from build123d import *

# Parameters (mm, degrees)
BOSS_EXTRU_1_DEPTH                             = 84
FRAISAGE_POUR_VIS_T_TE_FRAIS_E_M31_D           = 3.2
FRAISAGE_POUR_VIS_T_TE_FRAIS_E_M31_DEPTH       = 4
FRAISAGE_POUR_VIS_T_TE_FRAIS_E_M31_CSINK_D     = 6.3
FRAISAGE_POUR_VIS_T_TE_FRAIS_E_M31_CSINK_ANGLE = 90
D_GAGEMENT_M1_61_D                             = 1.7
D_GAGEMENT_M1_61_DEPTH                         = 4
ENL_V_MAT_EXTRU_1_DEPTH                        = 4
ENL_V_MAT_EXTRU_2_DEPTH                        = 31.75
ENL_V_MAT_EXTRU_2_DEPTH_BACK                   = 5


with BuildPart() as part:
    # Esquisse1 → Boss.-Extru.1 (new body)
    with BuildSketch(Plane.XY):
        with BuildLine():
            Line((0, 0), (-25, 0))
            ThreePointArc((-25, 0), (-32.071067812, 2.928932188), (-35, 10))
            Line((-35, 10), (-35, 45))
            Line((-35, 45), (-31, 45))
            Line((-31, 45), (-31, 10))
            ThreePointArc((-31, 10), (-29.242640687, 5.757359313), (-25, 4))
            Line((-25, 4), (0, 4))
            Line((0, 4), (0, 0))
        make_face()
    extrude(amount=BOSS_EXTRU_1_DEPTH)

    # Fraisage pour vis à tête fraisée M31
    with Locations(Plane(origin=(-31, 0, 0), x_dir=(0, 0, 1), z_dir=(1, 0, 0))):
        with Locations((4, -41), (80, -41)):
            CounterSinkHole(FRAISAGE_POUR_VIS_T_TE_FRAIS_E_M31_D / 2, FRAISAGE_POUR_VIS_T_TE_FRAIS_E_M31_CSINK_D / 2, depth=FRAISAGE_POUR_VIS_T_TE_FRAIS_E_M31_DEPTH, counter_sink_angle=FRAISAGE_POUR_VIS_T_TE_FRAIS_E_M31_CSINK_ANGLE)

    # Dégagement M1.61
    with Locations(Plane(origin=(0, 0, 0), x_dir=(-1, 0, 0), z_dir=(0, -1, 0))):
        with Locations((20.75, -21.5), (20.75, -62.5), (4.25, -62.5), (4.25, -21.5)):
            Hole(D_GAGEMENT_M1_61_D / 2, depth=D_GAGEMENT_M1_61_DEPTH)

    # Esquisse6 → Enlèv. mat.-Extru.1 (cut)
    with BuildSketch(Plane.XZ):
        with BuildLine():
            Line((-35, 17.5), (-3.25, 17.5))
            ThreePointArc((-3.25, 17.5), (-1.128679656, 18.378679656), (-0.25, 20.5))
            Line((-0.25, 20.5), (-0.25, 23.5))
            ThreePointArc((-0.25, 23.5), (-0.835786438, 24.914213562), (-2.25, 25.5))
            Line((-2.25, 25.5), (-3.750142858, 25.5))
            ThreePointArc((-3.750142858, 25.5), (-5.097923909, 25.180202649), (-6.15836042, 24.288990826))
            ThreePointArc((-6.15836042, 24.288990826), (-17.832822404, 23.171534919), (-17.754587156, 34.899094322))
            ThreePointArc((-17.754587156, 34.899094322), (-17.012643745, 35.911706018), (-16.75, 37.139256723))
            Line((-16.75, 37.139256723), (-16.75, 46.860743277))
            ThreePointArc((-16.75, 46.860743277), (-17.012643745, 48.088293982), (-17.754587156, 49.100905678))
            ThreePointArc((-17.754587156, 49.100905678), (-17.832822404, 60.828465081), (-6.15836042, 59.711009174))
            ThreePointArc((-6.15836042, 59.711009174), (-5.097923909, 58.819797351), (-3.750142858, 58.5))
            Line((-3.750142858, 58.5), (-2.25, 58.5))
            ThreePointArc((-2.25, 58.5), (-0.835786438, 59.085786438), (-0.25, 60.5))
            Line((-0.25, 60.5), (-0.25, 63.5))
            ThreePointArc((-0.25, 63.5), (-1.128679656, 65.621320344), (-3.25, 66.5))
            Line((-3.25, 66.5), (-35, 66.5))
            Line((-35, 66.5), (-35, 84))
            Line((-35, 84), (0, 84))
            Line((0, 84), (0, 0))
            Line((0, 0), (-35, 0))
            Line((-35, 0), (-35, 17.5))
        make_face()
        with BuildLine():
            Line((-18.75, 46), (-18.75, 38))
            ThreePointArc((-18.75, 38), (-20.75, 36), (-22.75, 38))
            Line((-22.75, 38), (-22.75, 46))
            ThreePointArc((-22.75, 46), (-20.75, 48), (-18.75, 46))
        make_face()
    extrude(amount=-ENL_V_MAT_EXTRU_1_DEPTH, mode=Mode.SUBTRACT)

    # Esquisse7 → Enlèv. mat.-Extru.2 (cut, two sides)
    with BuildSketch(Plane(origin=(-31, 0, 0), x_dir=(0, 0, -1), z_dir=(1, 0, 0))) as enl_v_mat_extru_2_sk:
        with BuildLine():
            Line((-60.518790495, 10), (-23.481209505, 10))
            Line((-23.481209505, 10), (-17.352509418, 22.636031611))
            ThreePointArc((-17.352509418, 22.636031611), (-17.875393601, 32.308498663), (-26.350052411, 37))
            Line((-26.350052411, 37), (-57.649947589, 37))
            ThreePointArc((-57.649947589, 37), (-66.124606399, 32.308498663), (-66.647490582, 22.636031611))
            Line((-66.647490582, 22.636031611), (-60.518790495, 10))
        make_face()
        with BuildLine():
            Line((-23.657740647, 9.636031611), (-23.481209505, 10))
            Line((-23.481209505, 10), (-60.518790495, 10))
            Line((-60.518790495, 10), (-60.342259353, 9.636031611))
            ThreePointArc((-60.342259353, 9.636031611), (-56.653215023, 5.52534119), (-51.34471636, 4))
            Line((-51.34471636, 4), (-32.65528364, 4))
            ThreePointArc((-32.65528364, 4), (-27.346784977, 5.52534119), (-23.657740647, 9.636031611))
        make_face()
        Polygon((0, 4), (0, 10), (-14.589893279, 10), (-17.5, 4), align=None)
        with BuildLine():
            Line((0, 10), (0, 41))
            ThreePointArc((0, 41), (-0.101534354, 40.104474676), (-0.400982803, 39.254412644))
            Line((-0.400982803, 39.254412644), (-14.589893279, 10))
            Line((-14.589893279, 10), (0, 10))
        make_face()
        with BuildLine():
            ThreePointArc((-4, 45), (-1.171572875, 43.828427125), (0, 41))
            Line((0, 41), (0, 45))
            Line((0, 45), (-4, 45))
        make_face()
        with BuildLine():
            ThreePointArc((-83.599017197, 39.254412644), (-83.898465646, 40.104474676), (-84, 41))
            Line((-84, 41), (-84, 10))
            Line((-84, 10), (-69.410106721, 10))
            Line((-69.410106721, 10), (-83.599017197, 39.254412644))
        make_face()
        Polygon((-69.410106721, 10), (-84, 10), (-84, 4), (-66.5, 4), align=None)
        with BuildLine():
            ThreePointArc((-84, 41), (-82.828427125, 43.828427125), (-80, 45))
            Line((-80, 45), (-84, 45))
            Line((-84, 45), (-84, 41))
        make_face()
    extrude(amount=ENL_V_MAT_EXTRU_2_DEPTH, mode=Mode.SUBTRACT)
    extrude(enl_v_mat_extru_2_sk.sketch, amount=-ENL_V_MAT_EXTRU_2_DEPTH_BACK, mode=Mode.SUBTRACT)


solid = part.part
Input: part model. Units: mm. Frame: model coordinates. A direction names the side the tool comes from. Coordinates: 2 decimals unless noted, no trailing zeros. Loops run counter-clockwise (first coordinate to the right, second up) from the corner with the lowest first, then second, coordinate; pieces in that order, holes last.
(1) First-contact query: pin 1 Ø1.2 at (y, z) = (1, 43.5) entering from -X; pin 2 Ø3.5 at (y, z) = (41, 80) entering from +X; pin 3 Ø16.5 at (x, z) = (-10.5, 30.5) entering from +Y. Flat tips, straight axial feed; report the tip coordinate or a pass-through.
(2) Section B-B on z = 30. Return the cut outline in (x, y), then the cut area to 3 significant figures.
(3) Section A-A on y = 31. Return the cut outline in (x, z), then the cut area to 3 significant figures.
(4) Material intervals for probe 1 along Z at (x, y) = (-20.75, 0.95); probe 2 along X at (y, z) = (39.5, 30.5); probe 3 along X at (y, z) = (3, 21), sorted ascending.
(5) Set-up query: faces 1 (the face through (-16.75, 2, 42)), 2 (the face through (-31, 2, 42)), 3 (the face through (-35, 39, 41)), 4 (the face through (-31.04, 4.9, 28.51)), 5 (the face through (-18.75, 2, 42)). Return all of +Z, -Z, +X, -X, +Y, -Y with unobstructed straight access to the full face (end or side cutting, diameter ignored); none if empty.
(6) Pull-direction query (Z, two-part tool) for faces 6 (the face through (-18, 2, 17.5)), 7 (the face through (-21.42, 2.03, 22.02)), 8 (the face through (-18, 0, 42)); classes: released by +Z, released by -Z, zero draft, split by the parting line, or undercut.
(7) Section C-C on x = -10. Return the cut outline in (y, z), then the cut area to 3 significant figures.
(8) Section D-D on x = -26.5. Return the cut outline in (y, z), then the cut area to 3 significant figures.
Data:
1. pin 1: stops at x = -30.43
1. pin 2: stops at x = -32.4
1. pin 3: stops at y = 4
2. outline: (-35, 37) - (-31, 37) - (-31, 45) - (-35, 45) - close; (-33.26, 4.36) arc R10 ccw to (-25, 0) - (-20.34, 0) - (-20.34, 4) - (-25, 4) arc R6 cw to (-27.04, 4.36) - close
2. area: 75.4 mm2
3. outline: (-35, 4.4) - (-31, 4.4) - (-31, 17.18) - (-35, 17.18) - close; (-35, 66.82) - (-31, 66.82) - (-31, 79.6) - (-35, 79.6) - close
3. area: 102 mm2
4. probe 1: z = 17.5 to 20.65, 22.35 to 36, 48 to 61.65, 63.35 to 66.5
4. probe 2: x = -35 to -31
4. probe 3: x = -32.14 to -21.44, -20.06 to -4.94, -3.56 to -0.25
5. face 1: +X, +Y, -Y
5. face 2: +Z, -Z, -X, -Y
5. face 3: +Z, -Z, -X, +Y, -Y
5. face 4: +X, -X
5. face 5: +Y, -Y
6. face 6: released by -Z
6. face 7: undercut
6. face 8: zero draft
7. outline: (0, 17.5) - (4, 17.5) - (4, 21.51) - (0, 21.51) - close; (0, 62.49) - (4, 62.49) - (4, 66.5) - (0, 66.5) - close
7. area: 32.0 mm2
8. outline: (0.11, 17.5) - (4, 17.5) - (4.19, 17.41) - (4.19, 30.71) arc R10 cw to (4, 32.66) - (4, 51.34) arc R10 cw to (4.19, 53.29) - (4.19, 66.59) - (4, 66.5) - (0.11, 66.5) - close
8. area: 196 mm2
